Work out the finished part from the listing and answer in its coordinate system (mm). A direction names the side the tool comes from. Coordinates: 2 decimals unless noted, no trailing zeros. Order: outer loops, then holes, each group sorted by start corner. A loop starts at its lowest first (then second) coordinate and runs counter-clockwise, first axis right, second up. Notation, with made-up numbers: (56.25, 42) -> (88.25, 42) arc R19 cw to (88.25, 54) -> close; hole circle Ø4 at (35, 14.25). An arc over 180 degrees is marked (long way). Write item = value, one per line. Start each with the question number.
Q1. The part is cut by section C-C, the plane z = 6. Determine the outline of the cut face in (x, y), plus the area to 3 significant figures.
Q2. The part is cut by section B-B, the plane y = 0. Determine the outline of the cut face in (x, z), plus the area to 3 significant figures.
Q3. Flat-ended cylindrical pins translate along their axes: pin 1 (2 mm diameter, centred on x = -5.5, y = 10.5, fed in from -Z); pin 2 (12 mm diameter, centred on y = 0, z = 49, fed in from -X); pin 3 (4.5 mm diameter, centred on x = 0, y = 0, fed in from -Z); pin 4 (1.2 mm diameter, centred on x = -0.5, y = -0.5, fed in from +Z). Find the tip coordinate at first contact, or state that the pin passes through.
Q4. The part is cut by section D-D, the plane y = -20. Determine the outline of the cut face in (x, z), plus the area to 3 significant figures.
Q5. For a pull along Z with two mould halves and no side action, classify faces 1 (the cylindrical face through (0, -2, 160)), 2 (the flat face through (0, 0, 155)), 3 (the cylindrical face through (-0.325, -0.105, 4.536)) as +Z half, -Z half, draft (parallel to the pull), parting line (faces both ways), or undercut.
Q6. The part is cut by section A-A, the plane x = 0. Determine the outline of the cut face in (y, z).
Q7. Straight lines are drawn through the part: L1, parallel to Y at x = 0, z = 157.75; L2, parallel to Z at x = 0, y = -3; L3, parallel to Z at x = 9, y = -3. For each, find the intervals that lie inside material, in ascending order. Write a range as from..to.
Q8. Which of the six approach directions +Z, -Z, +X, -X, +Y, -Y give full straight-line access (tool end or side, diameter ignored) to faces 4 (the flat face through (0, -5, 165)), 5 (the cylindrical face through (-7.493, 0.33, 78.88))?
```python
from build123d import *

# Parameters (mm, degrees)
F0_R          = 7.5
F1_DEPTH      = 160
F2_R          = 25
F3_DEPTH      = 5
F4_R          = 1.5
F5_DEPTH      = 7.5
F5_DEPTH_BACK = 7.5
F6_R          = 2
F7_DEPTH      = 10


with BuildPart() as f1:
    # F0 (on Top) → F1 (new body)
    with BuildSketch(Plane.XY):
        Circle(F0_R)
    extrude(amount=F1_DEPTH)

    # F2 (on face) → F3 (join)
    with BuildSketch(Plane.XY.offset(160)):
        Circle(F2_R)
    extrude(amount=F3_DEPTH)

    # F4 (on Front) → F5 (cut, two sides)
    with BuildSketch(Plane.XZ) as f5_sk:
        with Locations((0, 6)):
            Circle(F4_R)
    extrude(amount=-F5_DEPTH, mode=Mode.SUBTRACT)
    extrude(f5_sk.sketch, amount=F5_DEPTH_BACK, mode=Mode.SUBTRACT)

    # F6 (on face) → F7 (cut)
    with BuildSketch(Plane.XY.offset(165)):
        Circle(F6_R)
    extrude(amount=-F7_DEPTH, mode=Mode.SUBTRACT)


solid = f1.part
```
Model answer:
q1.outline = (-1.5, -7.35) -> (-1.5, 7.35) arc R7.5 ccw to start; (1.5, -7.35) arc R7.5 ccw to (1.5, 7.35) -> close
q1.area = 132 mm2
q2.outline = (-25, 160) -> (-7.5, 160) -> (-7.5, 0) -> (7.5, 0) -> (7.5, 160) -> (25, 160) -> (25, 165) -> (2, 165) -> (2, 155) -> (-2, 155) -> (-2, 165) -> (-25, 165) -> close; hole circle Ø3 at (0, 6)
q2.area = 2,600 mm2
q3.pin_1 = 160
q3.pin_2 = -7.5
q3.pin_3 = 0
q3.pin_4 = 155
q4.outline = (-15, 160) -> (15, 160) -> (15, 165) -> (-15, 165) -> close
q4.area = 150 mm2
q5.face_1 = draft
q5.face_2 = +Z half
q5.face_3 = undercut
q6.outline = (-25, 160) -> (-7.5, 160) -> (-7.5, 7.5) -> (7.5, 7.5) -> (7.5, 160) -> (25, 160) -> (25, 165) -> (2, 165) -> (2, 155) -> (-2, 155) -> (-2, 165) -> (-25, 165) -> close; (-7.5, 0) -> (7.5, 0) -> (7.5, 4.5) -> (-7.5, 4.5) -> close
q7.L1 = -7.5..-2, 2..7.5
q7.L2 = 0..4.5, 7.5..165
q7.L3 = 160..165
q8.face_4 = +Z, +X, -X, +Y, -Y
q8.face_5 = -Z
